```python
from build123d import *

# Parameters (mm, degrees)
CYLINDER007_R           = 6
CYLINDER007_DEPTH       = 236
CYLINDER007_PITCH_ANGLE = 90
CYLINDER006_R           = 10
CYLINDER006_DEPTH       = 10
CYLINDER006_PITCH_ANGLE = 90


with BuildPart() as connector_bore:
    # Cylinder007 → Cylinder007 (new body)
    with BuildSketch(Plane.XY):
        Circle(CYLINDER007_R)
    extrude(amount=CYLINDER007_DEPTH)


with BuildPart() as connector_bore_1:
    # Cylinder007 pitch: moved
    add(connector_bore.part.rotate(Axis((0, 0, 0), (0, 1, 0)), CYLINDER007_PITCH_ANGLE))


with BuildPart() as connector_bore_2:
    # Cylinder007 placement: moved
    add(connector_bore_1.part.moved(Location((-45, 0, 0))))


with BuildPart() as cut001:
    # Cylinder006 → Cylinder006 (new body)
    with BuildSketch(Plane.XY):
        Circle(CYLINDER006_R)
    extrude(amount=CYLINDER006_DEPTH)


with BuildPart() as cut001_1:
    # Cylinder006 pitch: moved
    add(cut001.part.rotate(Axis((0, 0, 0), (0, 1, 0)), CYLINDER006_PITCH_ANGLE))


with BuildPart() as cut001_2:
    # Cylinder006 placement: moved
    add(cut001_1.part.moved(Location((181, 0, 0))))

    # Cut001: cut connector_bore
    add(connector_bore_2.part, mode=Mode.SUBTRACT)


solid = cut001_2.part
```
Work out the finished part from the listing and answer in its coordinate system (mm). Give positions to 0.01 mm unless a question says otherwise; leave off trailing zeros. Order: outer loops, then holes, each group sorted by start corner. A loop starts at its lowest first (then second) coordinate and runs counter-clockwise, first axis right, second up. Notation, with made-up numbers: M 13.25,41.5 L 28.25,41.5 A33 ccw 28.25,78.5 Z; hole C 68.5,41 d3. An arc over 180 degrees is marked long. Return JSON: item names as keys, results as strings.
1) Section D-D, the plane y = 8.5 is taken. Write down the section's boundary in (x, z), plus the area to 3 significant figures.
Resolved:
{"outline": "M 181,-5.27 L 191,-5.27 L 191,5.27 L 181,5.27 Z", "area": "105 mm^2"}
2) Section A-A, the plane z = 0 is taken. Write down the section's boundary in (x, y).
Resolved:
{"outline": "M 181,-10 L 191,-10 L 191,-6 L 181,-6 Z; M 181,6 L 191,6 L 191,10 L 181,10 Z"}
3) Section C-C, the plane x = 184.75 is taken. Write down the section's boundary in (y, z).
Resolved:
{"outline": "C 0,0 d20; hole C 0,0 d12"}
4) Straight lines are drawn through the part: line 1 along Y through (x, z) = (184.5, 0); line 2 along Z through (x, y) = (185.5, 1.5); line 3 along Z through (x, y) = (186, -3). For each, find the intervals that lie inside material, in ascending order. Write a range as [from, to].
Resolved:
{"line 1": "[-10, -6], [6, 10]", "line 2": "[-9.89, -5.81], [5.81, 9.89]", "line 3": "[-9.54, -5.2], [5.2, 9.54]"}
5) Each of these flat-tipped pins is pushed along its axis until it touches: pin 1 (4 mm diameter, centred on x = 183.5, z = -5, fed in from -Y); pin 2 (1 mm diameter, centred on x = 184, y = -5.5, fed in from +Z); pin 3 (5 mm diameter, centred on x = 188.5, y = -5.5, fed in from +Z). Where does it stop, or does it pass through?
Resolved:
{"pin 1": "y = -9.54", "pin 2": "z = 8.66", "pin 3": "z = 9.54"}
6) For a pull along Z with two mould halves and no side action, classify faces 1 (the cylindrical face through (185.93, 1.802, -5.723)), 2 (the cylindrical face through (185.93, -9.76, 2.17)), 3 (the flat face through (191, -7, 0)) as +Z half, -Z half, draft (parallel to the pull), parting line (faces both ways), or undercut.
Resolved:
{"face 1": "undercut", "face 2": "parting line", "face 3": "draft"}
